from build123d import *

# Parameters (mm, degrees)
F3_R      = 75
F8_R      = 49.537672475
F13_DEPTH = 232


with BuildPart() as f4:
    # F4: sweep along a path in F0
    with BuildLine(Plane.XZ) as f4_path:
        Line((-350, 75), (-181.066017178, 75))
        ThreePointArc((-181.066017178, 75), (0, 0), (75, -181.066017178))
        Line((75, -181.066017178), (75, -350))
    # F3 (on plane+point) → F4 (sweep)
    with BuildSketch(Plane.YZ.offset(-350)):
        with Locations((0, 75)):
            Circle(F3_R)
    sweep(path=f4_path.line)

    # F8 (on plane+point) → F9 section 0
    with BuildSketch(Plane.YZ.offset(-1107.697725296)):
        with Locations((0, 75)):
            Circle(F8_R)
    # F3 (on plane+point) → F9 section 1
    with BuildSketch(Plane.YZ.offset(-350)):
        with Locations((0, 75)):
            Circle(F3_R)
    loft()

    # F10 (on Front) → F11 (revolve, cut)
    with BuildSketch(Plane.XZ):
        Polygon((-1085.869221311, 125.2712163399), (-1104.697725296, 124.6384870611), (-1099.2664424752, 113.0726968058), (-1090.5117942881, 113.3668955503), align=None)
        Polygon((-1060.530301493, 114.4205035296), (-1055.8877285158, 126.3248243192), (-1074.7162325009, 125.6920950404), (-1069.28494968, 114.1263047851), align=None)
        Polygon((-1030.5488086978, 115.4741115089), (-1025.9062357207, 127.3784322985), (-1044.7347397057, 126.7457030197), (-1039.3034568849, 115.1799127644), align=None)
        Polygon((-1000.5673159027, 116.5277194882), (-995.9247429255, 128.4320402778), (-1014.7532469106, 127.799310999), (-1009.3219640897, 116.2335207437), align=None)
        Polygon((-970.5858231075, 117.5813274675), (-965.9432501303, 129.4856482571), (-984.7717541154, 128.8529189783), (-979.3404712946, 117.287128723), align=None)
        Polygon((-940.6043303123, 118.6349354468), (-935.9617573352, 130.5392562364), (-954.7902613202, 129.9065269576), (-949.3589784994, 118.3407367023), align=None)
        Polygon((-910.6228375172, 119.6885434262), (-905.98026454, 131.5928642158), (-924.8087685251, 130.960134937), (-919.3774857043, 119.3943446816), align=None)
        Polygon((-880.641344722, 120.7421514055), (-875.9987717449, 132.6464721951), (-894.8272757299, 132.0137429163), (-889.3959929091, 120.447952661), align=None)
        Polygon((-850.6598519269, 121.7957593848), (-846.0172789497, 133.7000801744), (-864.8457829348, 133.0673508956), (-859.4145001139, 121.5015606403), align=None)
        Polygon((-820.6783591317, 122.8493673641), (-816.0357861546, 134.7536881537), (-834.8642901396, 134.1209588749), (-829.4330073188, 122.5551686196), align=None)
        Polygon((-790.6968663366, 123.9029753434), (-786.0542933594, 135.807296133), (-804.8827973445, 135.1745668542), (-799.4515145236, 123.6087765989), align=None)
        Polygon((-760.7153735414, 124.9565833227), (-756.0728005643, 136.8609041123), (-774.9013045493, 136.2281748335), (-769.4700217285, 124.6623845782), align=None)
        Polygon((-730.7338807463, 126.010191302), (-726.0913077691, 137.9145120916), (-744.9198117542, 137.2817828128), (-739.4885289333, 125.7159925575), align=None)
        Polygon((-700.7523879511, 127.0637992813), (-696.1098149739, 138.9681200709), (-714.938318959, 138.3353907921), (-709.5070361382, 126.7696005368), align=None)
        Polygon((-670.770895156, 128.1174072606), (-666.1283221788, 140.0217280502), (-684.9568261639, 139.3889987714), (-679.525543343, 127.8232085161), align=None)
        Polygon((-640.7894023608, 129.17101524), (-636.1468293836, 141.0753360296), (-654.9753333687, 140.4426067508), (-649.5440505479, 128.8768164954), align=None)
        Polygon((-610.8079095656, 130.2246232193), (-606.1653365885, 142.1289440089), (-624.9938405735, 141.4962147301), (-619.5625577527, 129.9304244747), align=None)
        Polygon((-580.8264167705, 131.2782311986), (-576.1838437933, 143.1825519882), (-595.0123477784, 142.5498227094), (-589.5810649575, 130.9840324541), align=None)
        Polygon((-550.8449239753, 132.3318391779), (-546.2023509982, 144.2361599675), (-565.0308549832, 143.6034306887), (-559.5995721624, 132.0376404334), align=None)
        Polygon((-520.8634311802, 133.3854471572), (-516.220858203, 145.2897679468), (-535.0493621881, 144.657038668), (-529.6180793672, 133.0912484127), align=None)
        Polygon((-490.881938385, 134.4390551365), (-486.2393654079, 146.3433759261), (-505.0678693929, 145.7106466473), (-499.6365865721, 134.144856392), align=None)
        Polygon((-460.9004455899, 135.4926631158), (-456.2578726127, 147.3969839054), (-475.0863765978, 146.7642546266), (-469.6550937769, 135.1984643713), align=None)
        Polygon((-430.9189527947, 136.5462710951), (-426.2763798176, 148.4505918847), (-445.1048838026, 147.8178626059), (-439.6736009818, 136.2520723506), align=None)
        Polygon((-400.9374599996, 137.5998790744), (-396.2948870224, 149.504199864), (-415.1233910075, 148.8714705852), (-409.6921081866, 137.3056803299), align=None)
        Polygon((-370.9559672044, 138.6534870538), (-366.3133942272, 150.5578078433), (-385.1418982123, 149.9250785646), (-379.7106153915, 138.3592883092), align=None)
    revolve(axis=Axis((-609.0528770564, 0, 75), (-1, 0, 0)), mode=Mode.SUBTRACT)

    # F12 (on Front) → F13 (cut, symmetric)
    with BuildSketch(Plane.XZ):
        Polygon((98.1314237101, 98.1314237101), (-114.6691401448, -114.6691401448), (-121.5471847165, -389.7904326519), (441.9294075858, -378.4590830407), align=None)
    extrude(amount=F13_DEPTH, both=True, mode=Mode.SUBTRACT)


solid = f4.part
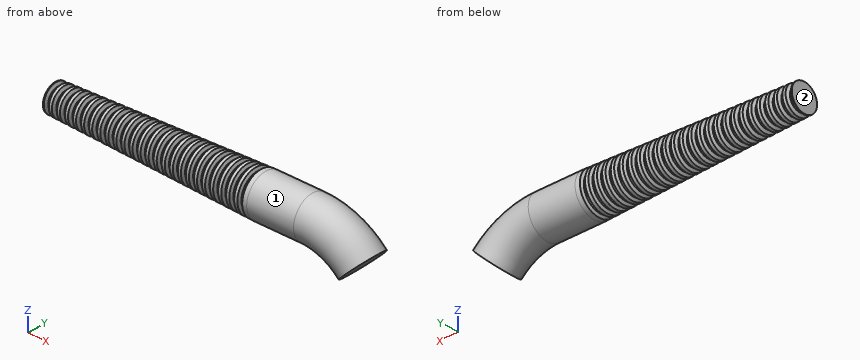
Geometry check sheet. Reference: the model listing, model coordinates, mm. Face numbers are marked on the shaded views. Give positions to 0.01 mm unless a question says otherwise; leave off trailing zeros. Loops run counter-clockwise (first coordinate to the right, second up) from the corner with the lowest first, then second, coordinate; pieces in that order, holes last.
(1) Depth check by flat-ended pin: pin 1 Ø10 at (y, z) = (21, 35.5) entering from +X; pin 2 Ø3 at (x, z) = (-720.5, 80.5) entering from -Y; pin 3 Ø1.5 at (x, z) = (-161, 10.5) entering from -Y. Enter the tip coordinate at first touch or a pass-through.
From the geometry:
pin 1: stops at x = 40.5
pin 2: stops at y = -62.43
pin 3: stops at y = -41.15
(2) Thickness scan on L1, parallel to X at y = -34, z = 54; L2, parallel to Y at x = -153, z = 116; L3, parallel to Z at x = -254.5, y = -15. Record the ranges inside material, lowest first.
From the geometry:
L1: x = -1107.7 to -1100.15, -1089.89 to -1069.68, -1060.32 to 40.34
L2: y = -61.92 to 61.92
L3: z = 1.52 to 148.48
(3) Release check for a two-part mould opening along Y. For the marked faces 1 and 2 record: released by +Y, released by -Y, zero draft, split by the parting line, or undercut.
From the geometry:
face 1: split by the parting line
face 2: zero draft
(4) Section check A-A on x = -205.5. Record the cut outline in (y, z).
From the geometry:
outline: circle Ø150 at (0, 75)
